Could you check a few things on this drawing? It's one solid part, dimensions in mm from its lowest x, y, z. A direction names the side the tool comes from. Round coordinates to 2 decimals unless told otherwise and drop trailing zeros. Write each loop counter-clockwise with the first axis right and the second up, starting at its lowest first coordinate (ties: lowest second). Pieces come first, ordered by that corner, then holes. Notation, with made-up numbers: (25.25, 5.5) - (55.25, 5.5) arc R18 cw to (55.25, 27.5) - close; hole circle Ø9 at (34, 45.5). An arc over 180 degrees is marked (long way). One line per question, with ' | ' between items. Start each with the question number.
(1) Imagine slicing it at B-B (y = 25.5). Write out the boundary of the cut face in (x, z).
(2) Imagine slicing it at C-C (x = 25.5). Write out the boundary of the cut face in (y, z).
(3) Imagine slicing it at D-D (z = 21.75). Write out the boundary of the cut face in (x, y), plus the area to 3 significant figures.
(4) Thinking about a two-plate mould opening in X: for the marked faces 3, 4 and 5, which applies, pulls with the +X half, pulls with the -X half, needs draft (parallel to the pull), parting line crosses it, or undercut?
(5) For the marked faces 1 and 2, which set-ups out of +Z, -Z, +X, -X, +Y, -Y let a thin tool reach every point of the face, with its end or its side?
(6) Will these pins go through, and if not, where does the flat tip stop? pin 1 (5 mm diameter, centred on x = 44, z = 4, fed in from -Y); pin 2 (2 mm diameter, centred on x = 34.5, y = 33.5, fed in from +Z); pin 3 (6 mm diameter, centred on x = 22.5, y = 33, fed in from +Z); pin 4 (8 mm diameter, centred on y = 44.5, z = 18.5, fed in from -X).
(7) Imagine slicing it at A-A (z = 14). Write out the boundary of the cut face in (x, y).
(8) If I drill on L1, parallel to Y at x = 8.5, z = 18.25; L2, parallel to Y at x = 41, z = 11.5; L3, parallel to X at y = 5.5, z = 24.75, over which ranges is the centre line in solid material (lowest first)?
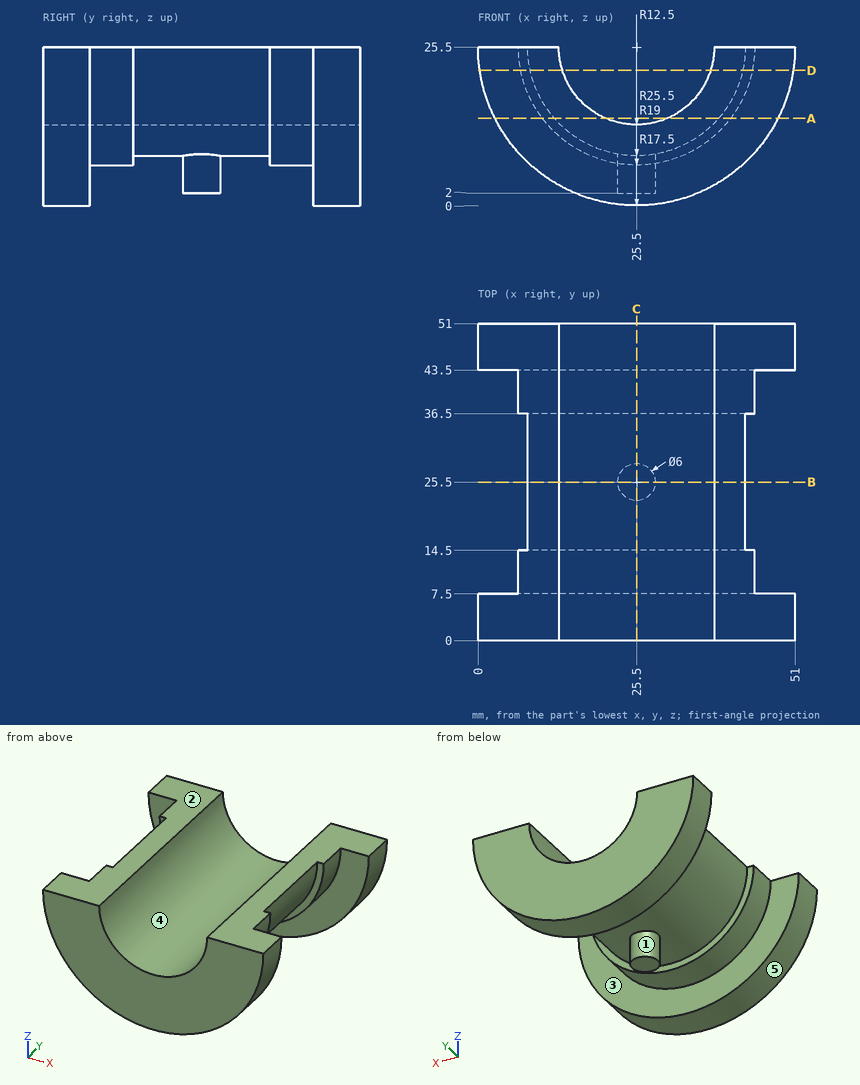
Check sheet entries:
1) outline: (8, 25.5) arc R17.5 ccw to (22.5, 8.26) - (22.5, 2) - (28.5, 2) - (28.5, 8.26) arc R17.5 ccw to (43, 25.5) - (38, 25.5) arc R12.5 cw to (13, 25.5) - close
2) outline: (0, 0) - (7.5, 0) - (7.5, 6.5) - (14.5, 6.5) - (14.5, 8) - (22.5, 8) - (22.5, 2) - (28.5, 2) - (28.5, 8) - (36.5, 8) - (36.5, 6.5) - (43.5, 6.5) - (43.5, 0) - (51, 0) - (51, 13) - (0, 13) - close
3) outline: (0.28, 0) - (13.58, 0) - (13.58, 51) - (0.28, 51) - (0.28, 43.5) - (6.87, 43.5) - (6.87, 36.5) - (8.41, 36.5) - (8.41, 14.5) - (6.87, 14.5) - (6.87, 7.5) - (0.28, 7.5) - close; (37.42, 0) - (50.72, 0) - (50.72, 7.5) - (44.13, 7.5) - (44.13, 14.5) - (42.59, 14.5) - (42.59, 36.5) - (44.13, 36.5) - (44.13, 43.5) - (50.72, 43.5) - (50.72, 51) - (37.42, 51) - close | area: 814 mm^2
4) face 3: needs draft | face 4: undercut | face 5: parting line crosses it
5) face 1: -Z | face 2: +Z, +X, -X, +Y, -Y
6) pin 1: through | pin 2: z = 18 | pin 3: z = 14.53 | pin 4: x = 0.18
7) outline: (2.74, 0) - (20.6, 0) - (20.6, 51) - (2.74, 51) - (2.74, 43.5) - (10.38, 43.5) - (10.38, 36.5) - (12.31, 36.5) - (12.31, 14.5) - (10.38, 14.5) - (10.38, 7.5) - (2.74, 7.5) - close; (30.4, 0) - (48.26, 0) - (48.26, 7.5) - (40.62, 7.5) - (40.62, 14.5) - (38.69, 14.5) - (38.69, 36.5) - (40.62, 36.5) - (40.62, 43.5) - (48.26, 43.5) - (48.26, 51) - (30.4, 51) - close
8) L1: 0 to 14.5, 36.5 to 51 | L2: 0 to 7.5, 43.5 to 51 | L3: 0.01 to 13.02, 37.98 to 50.99
